from build123d import *

# Parameters (mm, degrees)
F1_DEPTH = 63.5
F3_DEPTH = 12.7
F4_R     = 9.525
F5_DEPTH = 25.4
F6_W     = 19.05
F6_H     = 38.1
F7_DEPTH = 25.4
F8_W     = 19.05
F8_H     = 38.1
F9_DEPTH = 25.4
F10_R    = 6.35


with BuildPart() as f1:
    # F0 (on Top) → F1 (new body)
    with BuildSketch(Plane.XY):
        Polygon((-25.299002, 20.161893), (-37.999002, 20.161893), (-37.999002, -24.288107), (44.550998, -24.288107), (44.550998, -11.588107), (12.800998, -11.588107), (12.800998, 20.161893), (0.100998, 20.161893), (0.100998, -5.238107), (-25.299002, -5.238107), align=None)
    extrude(amount=F1_DEPTH)

    # F2 (on face) → F3 (join)
    with BuildSketch(Plane.XZ.offset(24.288107)):
        with BuildLine():
            Line((44.550998, 0), (44.550998, 63.5))
            ThreePointArc((44.550998, 63.5), (12.800998, 31.75), (44.550998, 0))
        make_face()
        with BuildLine():
            ThreePointArc((44.550998, 0), (67.001639, 9.29936), (76.300998, 31.75))
            ThreePointArc((76.300998, 31.75), (67.001639, 54.20064), (44.550998, 63.5))
            Line((44.550998, 63.5), (44.550998, 0))
        make_face()
    extrude(amount=-F3_DEPTH)

    # F4 (on face) → F5 (cut)
    with BuildSketch(Plane(origin=(0, -11.588107, 0), x_dir=(-1, 0, 0), z_dir=(0, 1, 0))):
        with Locations((-44.550998, 31.75)):
            Circle(F4_R)
    extrude(amount=-F5_DEPTH, mode=Mode.SUBTRACT)

    # F6 (on face) → F7 (cut)
    with BuildSketch(Plane.YZ.offset(12.800998)):
        with Locations((10.636893, 31.75)):
            Rectangle(F6_W, F6_H)
    extrude(amount=-F7_DEPTH, mode=Mode.SUBTRACT)

    # F8 (on face) → F9 (cut)
    with BuildSketch(Plane.YZ.offset(-25.299002)):
        with Locations((10.636893, 31.75)):
            Rectangle(F8_W, F8_H)
    extrude(amount=-F9_DEPTH, mode=Mode.SUBTRACT)

    # F10
    f10_edges = [f1.edges().sort_by_distance(p)[0] for p in [
        (12.800998, -11.588107, 31.75),
    ]]
    fillet(f10_edges, radius=F10_R)


solid = f1.part
Work out the finished part from the listing and answer in its coordinate system (mm). A direction names the side the tool comes from. Give positions to 0.01 mm unless a question says otherwise; leave off trailing zeros. Loops run counter-clockwise (first coordinate to the right, second up) from the corner with the lowest first, then second, coordinate; pieces in that order, holes last. Notation, with made-up numbers: (58, 70) -> (86, 70) arc R26 ccw to (86, 104) -> close; hole circle Ø10 at (39.5, 42). An arc over 180 degrees is marked (long way). Use a Markdown table: item, result. Add a question column.
1. Determine the mould class of faces 4 (the flat face through (-37.999, -7, 31)), 5 (the flat face through (-12, -5.238, 31)), 6 (the flat face through (7, 1.112, 31)) for opening direction X: released by +X, released by -X, zero draft, split by the parting line, or undercut.
2. Section C-C on y = 4.5 is taken. Determine the outline of the cut face in (x, z), and give its area (3 significant figures).
3. Section B-B on x = 9.5 is taken. Determine the outline of the cut face in (y, z).
4. Find the intervals of material crossed by probe 1 along Z at (x, y) = (-31.5, 17.5); probe 2 along X at (y, z) = (-3, 13); probe 3 along Y at (x, z) = (55, 34.5), in increasing order.
5. Flat-ended cylindrical pins translate along their axes: pin 1 Ø6.5 at (x, z) = (7.5, 24) entering from +Y; pin 2 Ø17 at (x, z) = (48, 42) entering from +Y; pin 3 Ø12.5 at (x, z) = (-17, 17) entering from +Y. Find the tip coordinate at first contact, or state that the pin passes through.
6. Section A-A on y = -4 is taken. Determine the outline of the cut face in (x, z), and give its area (3 significant figures).
7. Section D-D on x = 40.5 is taken. Determine the outline of the cut face in (y, z), and give its area (3 significant figures).
8. For faces 1 (the flat face through (0.101, -1, 31)), 2 (the flat face through (-32, 11, 12.7)), 3 (the flat face through (34.6, -11.588, 32.2)), determine the directions among +Z, -Z, +X, -X, +Y, -Y from which every point of the face is accessible in a straight line to the end or side of a thin tool.
Results below:
| question | item | result |
|---|---|---|
| 1 | face 4 | released by -X |
| 1 | face 5 | undercut |
| 1 | face 6 | zero draft |
| 2 | outline | (-38, 0) -> (-25.3, 0) -> (-25.3, 12.7) -> (-38, 12.7) -> close; (-38, 50.8) -> (-25.3, 50.8) -> (-25.3, 63.5) -> (-38, 63.5) -> close; (0.1, 0) -> (12.8, 0) -> (12.8, 12.7) -> (0.1, 12.7) -> close; (0.1, 50.8) -> (12.8, 50.8) -> (12.8, 63.5) -> (0.1, 63.5) -> close |
| 2 | area | 645 mm^2 |
| 3 | outline | (-24.29, 0) -> (20.16, 0) -> (20.16, 12.7) -> (1.11, 12.7) -> (1.11, 50.8) -> (20.16, 50.8) -> (20.16, 63.5) -> (-24.29, 63.5) -> close |
| 4 | probe 1 | z = 0 to 12.7, 50.8 to 63.5 |
| 4 | probe 2 | x = -38 to -25.3, 0.1 to 12.8 |
| 4 | probe 3 | y = -24.29 to -11.59 |
| 5 | pin 1 | stops at y = 1.11 |
| 5 | pin 2 | stops at y = -11.59 |
| 5 | pin 3 | stops at y = -5.24 |
| 6 | outline | (-38, 0) -> (-25.3, 0) -> (-25.3, 63.5) -> (-38, 63.5) -> close; (0.1, 0) -> (12.8, 0) -> (12.8, 63.5) -> (0.1, 63.5) -> close |
| 6 | area | 1,610 mm^2 |
| 7 | outline | (-24.29, 0) -> (-11.59, 0) -> (-11.59, 23.13) -> (-24.29, 23.13) -> close; (-24.29, 40.37) -> (-11.59, 40.37) -> (-11.59, 63.5) -> (-24.29, 63.5) -> close |
| 7 | area | 587 mm^2 |
| 8 | face 1 | +Z, -Z, +Y |
| 8 | face 2 | +X, -X, +Y |
| 8 | face 3 | +Z, -Z, +X, +Y |
